The listing builds one solid part. Answer for the finished solid, in the listing's coordinates (mm). A direction names the side the tool comes from. Give positions to 0.01 mm unless a question says otherwise; leave off trailing zeros. Order: outer loops, then holes, each group sorted by start corner. A loop starts at its lowest first (then second) coordinate and runs counter-clockwise, first axis right, second up. Notation, with made-up numbers: (43, -35) -> (59, -35) arc R18 ccw to (59, -16) -> close; hole circle Ø7 at (70, 60). An arc over 180 degrees is marked (long way). Answer as a JSON object with one key per item and string values. Group by question number.
```python
from build123d import *

# Parameters (mm, degrees)
F3_DEPTH = 25.4
F5_D     = 6.35


with BuildPart() as f1:
    # F0 (on Front) → F1 (revolve)
    with BuildSketch(Plane.XZ):
        with BuildLine():
            Line((82.624230206, 38.012702018), (-44.375769794, 38.012702018))
            Line((-44.375769794, 38.012702018), (-44.375769794, 36.3112246461))
            ThreePointArc((-44.375769794, 36.3112246461), (-39.7272471659, 31.662702018), (-38.025769794, 25.312702018))
            Line((-38.025769794, 25.312702018), (82.624230206, 25.312702018))
            Line((82.624230206, 25.312702018), (82.624230206, 31.662702018))
            Line((82.624230206, 31.662702018), (82.624230206, 38.012702018))
        make_face()
    revolve(axis=Axis((15.949230206, 0, 25.312702018), (-1, 0, 0)))

    # F2 (on face) → F3 (join)
    with BuildSketch(Plane.YZ.offset(82.624230206)):
        with BuildLine():
            Line((0, 25.3868182957), (0, 31.7368182957))
            Line((0, 31.7368182957), (-10.9553973023, 31.7368182957))
            ThreePointArc((-10.9553973023, 31.7368182957), (-12.2463268947, 28.6768479108), (-12.6997837296, 25.3868182957))
            Line((-12.6997837296, 25.3868182957), (0, 25.3868182957))
        make_face()
        with BuildLine():
            Line((0, 19.0368182957), (0, 25.3868182957))
            Line((0, 25.3868182957), (-12.6997837296, 25.3868182957))
            ThreePointArc((-12.6997837296, 25.3868182957), (-12.2876610608, 22.1028132887), (-11.0409819991, 19.0368182957))
            Line((-11.0409819991, 19.0368182957), (0, 19.0368182957))
        make_face()
        with BuildLine():
            Line((10.9553973023, 31.7368182957), (0, 31.7368182957))
            Line((0, 31.7368182957), (0, 25.3868182957))
            Line((0, 25.3868182957), (0, 19.0368182957))
            Line((0, 19.0368182957), (11.0409819991, 19.0368182957))
            ThreePointArc((11.0409819991, 19.0368182957), (12.2782423699, 22.0669718527), (12.7, 25.312702018))
            ThreePointArc((12.7, 25.312702018), (12.2560912558, 28.6410990993), (10.9553973023, 31.7368182957))
        make_face()
    extrude(amount=F3_DEPTH)

    # F5 (through all)
    with Locations(Plane(origin=(0, 0, 19.0368182957), x_dir=(1, 0, 0), z_dir=(0, 0, -1))):
        with Locations((101.674230206, 0)):
            Hole(F5_D / 2)


solid = f1.part
```
(1) A cutting plane is placed at C-C (y = -6). Determine the outline of the cut face in (x, z), and give its area (3 significant figures).
(2) Which of the six approach directions +Z, -Z, +X, -X, +Y, -Y give full straight-line access (tool end or side, diameter ignored) to faces 1 (the flat face through (95, 0, 19.037)), 2 (the flat face through (108.024, 0, 25)), 3 (the flat face through (82.624, 0, 34))?
(3) A cutting plane is placed at D-D (x = -30). Determine the outline of the cut face in (y, z), and give its area (3 significant figures).
(4) Find the intervals of material crossed by line 1 along X through (y, z) = (-9.5, 17.5); line 2 along X through (y, z) = (2.5, 22.25); line 3 along Z through (x, y) = (75, 0), in increasing order. Write a range as [from, to].
(5) For a pull along Y with two mould halves and no side action, classify faces 4 (the cylindrical face through (98.646, -0.954, 25.476)), 5 (the flat face through (-44.376, 11.3, 25.3)) as +Y half, -Y half, draft (parallel to the pull), parting line (faces both ways), or undercut.
(6) A cutting plane is placed at A-A (y = 0). Determine the outline of the cut face in (x, z).
(7) A cutting plane is placed at B-B (z = 22.5). Determine the outline of the cut face in (x, y) (3 decimals).
(8) Flat-ended cylindrical pins translate along their axes: pin 1 Ø5 at (y, z) = (-5, 36) entering from +X; pin 2 Ø6.5 at (x, y) = (101, 0) entering from +Z; pin 3 Ø1 at (x, y) = (44.5, -9.5) entering from -Z. Find the tip coordinate at first contact, or state that the pin passes through.
Check sheet entries:
{
 "1": {"outline": "(-44.38, 14.12) -> (82.62, 14.12) -> (82.62, 19.04) -> (108.02, 19.04) -> (108.02, 31.74) -> (82.62, 31.74) -> (82.62, 36.51) -> (-44.38, 36.51) -> (-44.38, 34.53) arc R11.19 cw to (-44.38, 16.09) -> close", "area": "3,100 mm2"},
 "2": {"face 1": "-Z, +X, +Y, -Y", "face 2": "+Z, -Z, +X, +Y, -Y", "face 3": "+Z, +X, +Y, -Y"},
 "3": {"outline": "circle Ø25.4 at (0, 25.31)", "area": "507 mm2"},
 "4": {"line 1": "x = [-44.38, 82.62]", "line 2": "x = [-38.66, 99.72], [103.63, 108.02]", "line 3": "z = [12.61, 38.01]"},
 "5": {"face 4": "undercut", "face 5": "draft"},
 "6": {"outline": "(-44.38, 12.61) -> (82.62, 12.61) -> (82.62, 19.04) -> (98.5, 19.04) -> (98.5, 31.74) -> (82.62, 31.74) -> (82.62, 38.01) -> (-44.38, 38.01) -> (-44.38, 36.31) arc R12.7 cw to (-44.38, 14.31) -> close; (104.85, 19.04) -> (108.02, 19.04) -> (108.02, 31.74) -> (104.85, 31.74) -> close"},
 "7": {"outline": "(-44.376, -12.385) -> (108.024, -12.385) -> (108.024, 12.385) -> (-44.376, 12.385) -> (-44.376, 10.633) arc R12.385 cw to (-44.376, -10.633) -> close; hole circle Ø6.35 at (101.674, 0)"},
 "8": {"pin 1": "stops at x = 82.62", "pin 2": "stops at z = 31.74", "pin 3": "stops at z = 16.35"}
}
